Part model, mm, in its own coordinate system. Face numbers are marked on the shaded views. Coordinates: 2 decimals unless noted, no trailing zeros. Order: outer loops, then holes, each group sorted by start corner. A loop starts at its lowest first (then second) coordinate and runs counter-clockwise, first axis right, second up.
1) Wall check: L1, parallel to X at y = 0.25, z = 0.45; L2, parallel to X at y = -0.5, z = 1.5; L3, parallel to Y at x = 1.5, z = 1.25. Give the ranges that are in metal, low to high.
2) Mould opens along Y. For the marked faces 1, 2 and 3 say: +Y half, -Y half, draft (parallel to the pull), parting line (faces both ways), or undercut.
3) Cut at A-A (z = 0.8). List the corners of the cut face in (x, y), and give its area (3 significant figures).
```python
from build123d import *

# Parameters (mm, degrees)
SKETCH1_R           = 2
BOSS_EXTRUDE1_DEPTH = 3.1
CHAMFER1_SIZE       = 0.35


with BuildPart() as part:
    # Sketch1 → Boss-Extrude1 (new body)
    with BuildSketch(Plane.XY):
        Polygon((3.45, 1.991858429), (0, 3.983716857), (-3.45, 1.991858429), (-3.45, -1.991858429), (0, -3.983716857), (3.45, -1.991858429), align=None)
        Circle(SKETCH1_R, mode=Mode.SUBTRACT)
    extrude(amount=BOSS_EXTRUDE1_DEPTH)

    # Chamfer1
    chamfer1_edges = [part.edges().sort_by_distance(p)[0] for p in [
        (-2, 0, 0),
        (-2, 0, 3.1),
    ]]
    chamfer(chamfer1_edges, length=CHAMFER1_SIZE)

    # Sketch2 → Cut-Revolve1 (revolve, cut)
    with BuildSketch(Plane(origin=(0, 0, 0), x_dir=(1, 0, 0), z_dir=(0, 1, 0))):
        with BuildLine():
            Line((-4, -0.3), (-4.500819954, -0.3))
            Line((-4.500819954, -0.3), (-4.500819954, 0.361239255))
            Line((-4.500819954, 0.361239255), (-3.45, 0.361239255))
            Line((-3.45, 0.361239255), (-3.45, 0))
            ThreePointArc((-3.45, 0), (-3.763249102, -0.079876646), (-4, -0.3))
        make_face()
        with BuildLine():
            Line((-3.45, -3.461239255), (-3.45, -3.1))
            ThreePointArc((-3.45, -3.1), (-3.763249102, -3.020123354), (-4, -2.8))
            Line((-4, -2.8), (-4.500819954, -2.8))
            Line((-4.500819954, -2.8), (-4.500819954, -3.461239255))
            Line((-4.500819954, -3.461239255), (-3.45, -3.461239255))
        make_face()
    revolve(axis=Axis((0, 0, 1.55), (0, 0, -1)), mode=Mode.SUBTRACT)


solid = part.part
```
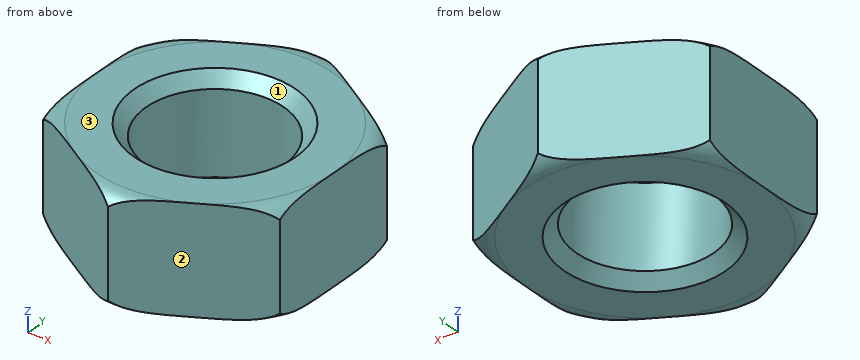
Geometry check:
1. L1: x = -3.45 to -1.98, 1.98 to 3.45
1. L2: x = -3.45 to -1.94, 1.94 to 3.45
1. L3: y = -3.12 to -1.32, 1.32 to 3.12
2. face 1: undercut
2. face 2: -Y half
2. face 3: draft
3. outline: (-3.45, -1.99) - (0, -3.98) - (3.45, -1.99) - (3.45, 1.99) - (0, 3.98) - (-3.45, 1.99) - close; hole circle Ø4 at (0, 0)
3. area: 28.7 mm2
